Autodesk Inventor part; units mm, degrees
ref_plane "YZ Plane" through (0, 0, 0) normal (1, 0, 0) x (0, 1, 0)
ref_plane "XZ Plane" through (0, 0, 0) normal (0, 1, 0) x (-1, 0, 0)
ref_plane "XY Plane" through (0, 0, 0) normal (0, 0, 1) x (1, 0, 0)
sketch "Boceto1" plane through (0, 0, 0) normal (0, 1, 0) x (-1, 0, 0)
  line L0 (0, 0) -> (-80, 0)
  line L1 (-80, 0) -> (-80, -40)
  line L2 (-80, -40) -> (0, -40)
  line L3 (0, -40) -> (0, 0)
  line L4 (-10, 0) -> (-70, 0)
  line L5 (-70, 0) -> (-70, -30)
  line L6 (-70, -30) -> (-10, -30)
  line L7 (-10, -30) -> (-10, 0)
  dimension "d0" = 80
  dimension "d1" = 40
  dimension "d2" = 60
  dimension "d3" = 30
extrude "Extrusión1" add sketch "Boceto1" along normal blind 150 contours L3 L2 L1 L0 L5 L6 L7
sketch "Boceto2" plane through (80, 0, -40) normal (0, 0, -1) x (-1, 0, 0)
  circle A0 centre (40, 120) radius 10
  circle A1 centre (40, 30) radius 10
  line L0 (0, 0) -> (80, 0)
  line L1 (80, 0) -> (80, 150)
  circle A2 centre (40, 75) radius 12.5
  dimension "d6" = 20
  dimension "d7" = 20
  dimension "d8" = 120
  dimension "d9" = 40
  dimension "d10" = 40
  dimension "d11" = 25
  dimension "d12" = 40
  dimension "d13" = 75
  dimension "d14" = 30
extrude "Extrusión2" cut sketch "Boceto2" against normal blind 150
properties part number "anclaje"
Geometry check sheet. Reference: the model listing, model coordinates, mm. A direction names the side the tool comes from. Coordinates: 2 decimals unless noted, no trailing zeros. Order: outer loops, then holes, each group sorted by start corner. A loop starts at its lowest first (then second) coordinate and runs counter-clockwise, first axis right, second up. Notation, with made-up numbers: (-5.75, 79.5) - (45.25, 79.5) arc R19 ccw to (45.25, 99.5) - close; hole circle Ø3 at (3.25, 69). An arc over 180 degrees is marked (long way). Answer in a Markdown table with one row per item. Add a question column.
1. Access from +Z, -Z, +X, -X, +Y, -Y to the whole of each face (thin tool, end or side, straight path). Record for faces 4 (the face through (10, 74, -15)), 5 (the face through (41.627, 87.394, -35.07)).
2. Section check C-C (y = 42). Enter the section's corners in (x, z), plus the area to 3 significant figures.
3. Gauge pin test, flat end, axial feed: pin 1 Ø6 at (x, y) = (34.5, 36) entering from +Z. Record the tip position at first contact, or that the pin passes through.
4. Section check B-B (z = -20.5). Enter the section's corners in (x, y).
5. Material ranges on L1, parallel to Y at x = 40, z = -33.25; L2, parallel to X at y = 56.5, z = -4; L3, parallel to Z at x = 29, y = 68.5, recorded low to high. Write a range as [from, to].
6. Section check A-A (x = 40). Enter the section's corners in (y, z).
7. Section check D-D (y = 120). Enter the section's corners in (x, z), plus the area to 3 significant figures.
8. Draft check along X on faces 1 (the face through (42.17, 20.24, -35.07)), 2 (the face through (80, 74, -20)), 3 (the face through (75, 74, 0)). Enter one of: +X half, -X half, draft (parallel to the pull), parting line (faces both ways), or undercut.
Data:
| question | item | result |
|---|---|---|
| 1 | face 4 | +Z, +Y, -Y |
| 1 | face 5 | +Z, -Z |
| 2 | outline | (0, -40) - (80, -40) - (80, 0) - (70, 0) - (70, -30) - (10, -30) - (10, 0) - (0, 0) - close |
| 2 | area | 1,400 mm² |
| 3 | pin 1 | stops at z = -30 |
| 4 | outline | (0, 0) - (10, 0) - (10, 150) - (0, 150) - close; (70, 0) - (80, 0) - (80, 150) - (70, 150) - close |
| 5 | L1 | y = [0, 20], [40, 62.5], [87.5, 110], [130, 150] |
| 5 | L2 | x = [0, 10], [70, 80] |
| 5 | L3 | z = [-40, -30] |
| 6 | outline | (0, -40) - (20, -40) - (20, -30) - (0, -30) - close; (40, -40) - (62.5, -40) - (62.5, -30) - (40, -30) - close; (87.5, -40) - (110, -40) - (110, -30) - (87.5, -30) - close; (130, -40) - (150, -40) - (150, -30) - (130, -30) - close |
| 7 | outline | (0, -40) - (30, -40) - (30, -30) - (10, -30) - (10, 0) - (0, 0) - close; (50, -40) - (80, -40) - (80, 0) - (70, 0) - (70, -30) - (50, -30) - close |
| 7 | area | 1,200 mm² |
| 8 | face 1 | undercut |
| 8 | face 2 | +X half |
| 8 | face 3 | draft |
